The model under review builds one solid part; all positions refer to its coordinate system, in mm. Round coordinates to 2 decimals unless told otherwise and drop trailing zeros. Loops run counter-clockwise (first coordinate to the right, second up) from the corner with the lowest first, then second, coordinate; pieces in that order, holes last. Notation, with made-up numbers: (1.25, 46) - (32.25, 46) arc R20 ccw to (32.25, 70) - close; hole circle Ø10 at (-25, 68.25). An arc over 180 degrees is marked (long way). Answer as CSV lines item,"result".
from build123d import *

# Parameters (mm, degrees)
SKETCH_1_R      = 2.6
SKETCH_1_W      = 15
SKETCH_1_H      = 15
EXTRUDE_1_DEPTH = 2


with BuildPart() as part:
    # 草图1 → 凸台-拉伸1 (new body)
    # profile 1 of 2: a face of its own
    with BuildSketch(Plane.XY):
        Polygon((0, 17.5), (0, 0), (15, 0), (15, 2.5), (31.1, 2.5), (31.1, 17.5), align=None)
        with Locations((7.5, 7.5)):
            Circle(SKETCH_1_R, mode=Mode.SUBTRACT)
        with BuildLine():
            ThreePointArc((17.1, 7.9), (15, 10), (17.1, 12.1))
            Line((17.1, 12.1), (25.1, 12.1))
            ThreePointArc((25.1, 12.1), (27.2, 10), (25.1, 7.9))
            Line((25.1, 7.9), (17.1, 7.9))
        make_face(mode=Mode.SUBTRACT)
    # profile 2 of 2: a face of its own
    with BuildSketch(Plane.XY):
        with Locations((7.5, -7.5)):
            Rectangle(SKETCH_1_W, SKETCH_1_H)
        with Locations((7.5, -7.5)):
            Circle(SKETCH_1_R, mode=Mode.SUBTRACT)
    extrude(amount=EXTRUDE_1_DEPTH)


solid = part.part
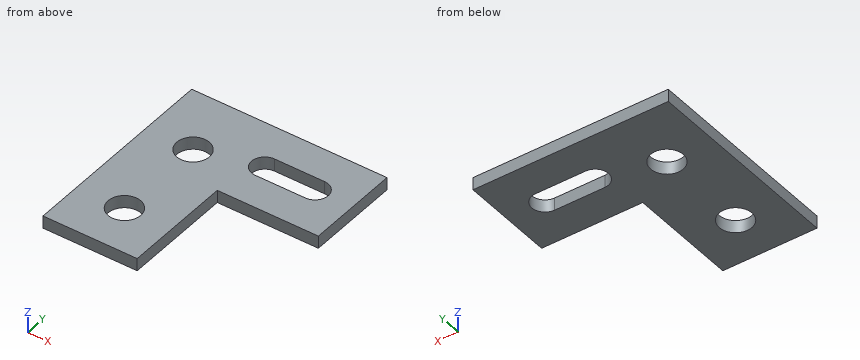
1. Take a section at A-A (y = 7.5). State the section outline as (x, z) points.
Numbers:
outline,"(0, 0) - (4.9, 0) - (4.9, 2) - (0, 2) - close; (10.1, 0) - (31.1, 0) - (31.1, 2) - (10.1, 2) - close"
2. Clearance check with flat-ended pins moving along their axes: pin 1 (1 mm diameter, centred on x = 21.5, z = 1.5, fed in from -Y); pin 2 (6 mm diameter, centred on x = 4.5, y = -10, fed in from -Z); pin 3 (0.6 mm diameter, centred on y = -5.5, z = 1, fed in from +X). State where each tip first meets the part, or that it passes through.
Numbers:
pin 1,"stops at y = 2.5"
pin 2,"stops at z = 0"
pin 3,"stops at x = 15"
3. Wall thickness on probe 1 along Y at (x, z) = (7.5, 1.65); probe 2 along Y at (x, z) = (25, 1.3); probe 3 along X at (y, z) = (9, 0.2): over which ranges is each line inside the solid? List them lowest first.
Numbers:
probe 1,"y = -15 to -10.1, -4.9 to 4.9, 10.1 to 17.5"
probe 2,"y = 2.5 to 7.9, 12.1 to 17.5"
probe 3,"x = 0 to 5.38, 9.62 to 15.25, 26.95 to 31.1"
4. Take a section at B-B (x = 7.5). State the section outline as (y, z) points.
Numbers:
outline,"(-15, 0) - (-10.1, 0) - (-10.1, 2) - (-15, 2) - close; (-4.9, 0) - (4.9, 0) - (4.9, 2) - (-4.9, 2) - close; (10.1, 0) - (17.5, 0) - (17.5, 2) - (10.1, 2) - close"
5. Take a section at D-D (x = 16.5). State the section outline as (y, z) points, plus the area to 3 significant figures.
Numbers:
outline,"(2.5, 0) - (7.99, 0) - (7.99, 2) - (2.5, 2) - close; (12.01, 0) - (17.5, 0) - (17.5, 2) - (12.01, 2) - close"
area,"22.0 mm²"
6. Take a section at C-C (z = 1.1). State the section outline as (x, y) points.
Numbers:
outline,"(0, -15) - (15, -15) - (15, 2.5) - (31.1, 2.5) - (31.1, 17.5) - (0, 17.5) - close; hole circle Ø5.2 at (7.5, -7.5); hole circle Ø5.2 at (7.5, 7.5); hole (17.1, 7.9) - (25.1, 7.9) arc R2.1 ccw to (25.1, 12.1) - (17.1, 12.1) arc R2.1 ccw to start"
